Drawing for the job (mm, zero at the part's lowest x, y, z). Round coordinates to 2 decimals unless told otherwise and drop trailing zeros. Loops run counter-clockwise (first coordinate to the right, second up) from the corner with the lowest first, then second, coordinate; pieces in that order, holes last. Notation, with made-up numbers: M 56.5,77 L 72.5,77 A17 ccw 72.5,101 Z; hole C -33.75,65 d7. An arc over 180 degrees is marked long. Answer in a Markdown table with one row per item.
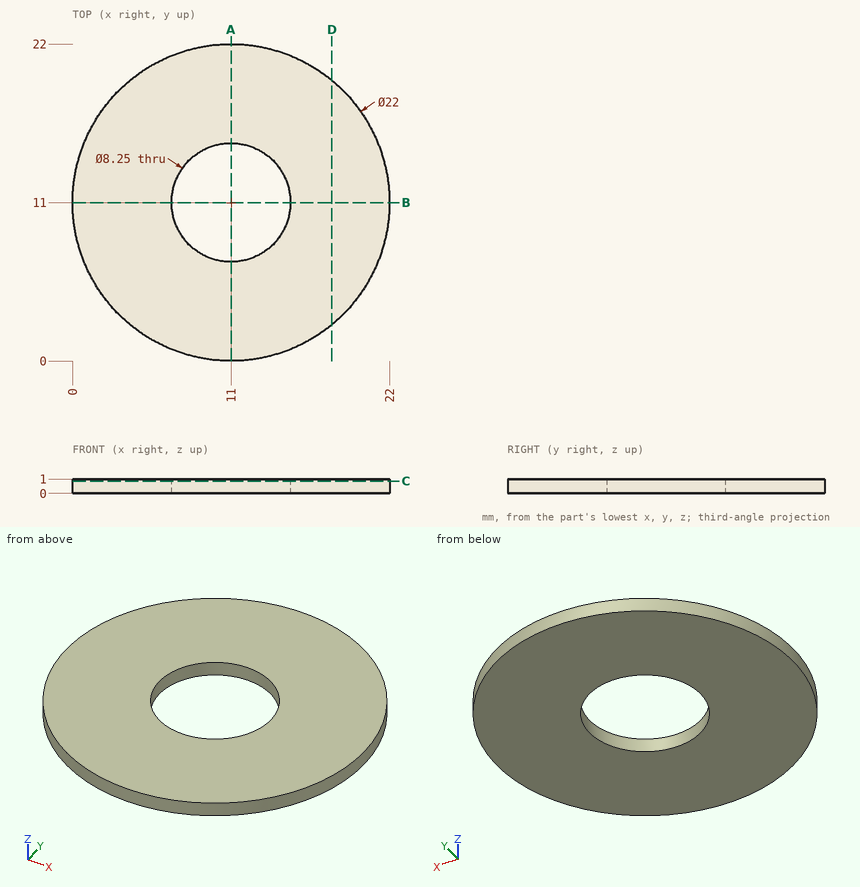
1. Saw through at C-C (z = 0.85). Write the cut outline in (x, y) (3 decimals).
Verdict:
| item | result |
|---|---|
| outline | C 11,11 d22; hole C 11,11 d8.25 |
2. Saw through at D-D (x = 18). Write the cut outline in (y, z), and give its area (3 significant figures).
Verdict:
| item | result |
|---|---|
| outline | M 2.51,0 L 19.49,0 L 19.49,1 L 2.51,1 Z |
| area | 17.0 mm² |
3. Saw through at A-A (x = 11). Write the cut outline in (y, z) (3 decimals).
Verdict:
| item | result |
|---|---|
| outline | M 0,0 L 6.875,0 L 6.875,1 L 0,1 Z; M 15.125,0 L 22,0 L 22,1 L 15.125,1 Z |
4. Wall check: probe 1 along Y at (x, z) = (11, 0.4) (3 decimals); probe 2 along X at (y, z) = (14, 0.4); probe 3 along Y at (x, z) = (7.5, 0.9). Give the ranges that are in metal, low to high.
Verdict:
| item | result |
|---|---|
| probe 1 | y = 0 to 6.875, 15.125 to 22 |
| probe 2 | x = 0.42 to 8.17, 13.83 to 21.58 |
| probe 3 | y = 0.57 to 8.82, 13.18 to 21.43 |
